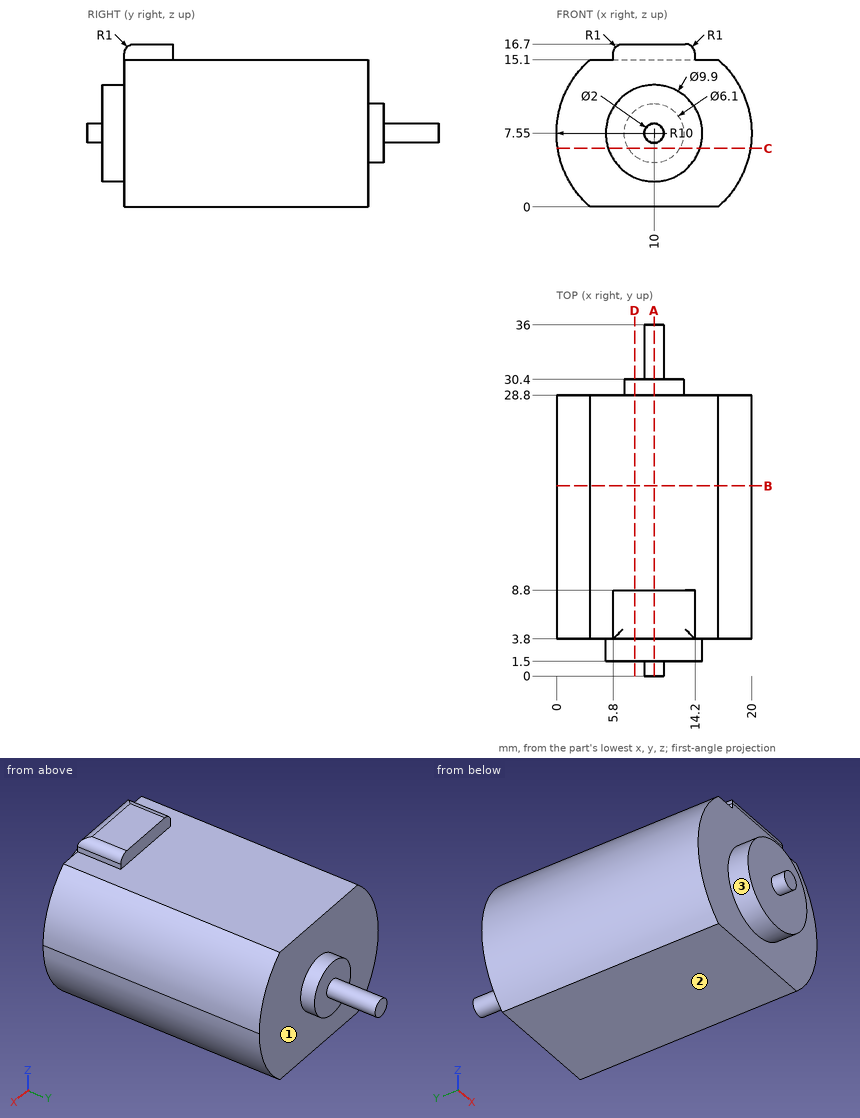
Print and shaded views of the part. All mm, measured from the part's lowest x, y and z. A direction names the side the tool comes from. Give positions to 0.01 mm unless a question says otherwise; leave off trailing zeros. Loops run counter-clockwise (first coordinate to the right, second up) from the corner with the lowest first, then second, coordinate; pieces in that order, holes last. Notation, with made-up numbers: (88.5, 34) -> (100.5, 34) arc R18 ccw to (100.5, 67) -> close; hole circle Ø3 at (28, 72). An arc over 180 degrees is marked (long way). Use a Markdown table: item, result.
1. Wall check: L1, parallel to Y at x = 6.25, z = 14.25; L2, parallel to X at y = 35.5, z = 7.5; L3, parallel to Z at x = 7.75, y = 25.5. Give the ranges that are in metal, low to high. Write a range as [from, to].
Check result:
| item | result |
|---|---|
| L1 | y = [3.8, 28.8] |
| L2 | x = [9, 11] |
| L3 | z = [0, 15.1] |
2. Which spindle directions (+Z, -Z, +X, -X, +Y, -Y) get a long thin tool onto all of the face, cutting with end or side? Do the marked faces 1, 2 and 3. Say none if no direction does.
Check result:
| item | result |
|---|---|
| face 1 | +Y |
| face 2 | -Z, +X, -X, +Y, -Y |
| face 3 | -Y |
3. Slice it at C-C (z = 6). List the corners of the cut face in (x, y), plus the area to 3 significant figures.
Check result:
| item | result |
|---|---|
| outline | (0.12, 3.8) -> (5.3, 3.8) -> (5.3, 1.5) -> (14.7, 1.5) -> (14.7, 3.8) -> (19.88, 3.8) -> (19.88, 28.8) -> (12.63, 28.8) -> (12.63, 30.4) -> (7.37, 30.4) -> (7.37, 28.8) -> (0.12, 28.8) -> close |
| area | 524 mm^2 |
4. Slice it at A-A (x = 10). List the corners of the cut face in (y, z).
Check result:
| item | result |
|---|---|
| outline | (0, 6.55) -> (1.5, 6.55) -> (1.5, 2.6) -> (3.8, 2.6) -> (3.8, 0) -> (28.8, 0) -> (28.8, 4.5) -> (30.4, 4.5) -> (30.4, 6.55) -> (36, 6.55) -> (36, 8.55) -> (30.4, 8.55) -> (30.4, 10.6) -> (28.8, 10.6) -> (28.8, 15.1) -> (8.8, 15.1) -> (8.8, 16.7) -> (4.8, 16.7) arc R1 ccw to (3.8, 15.7) -> (3.8, 12.5) -> (1.5, 12.5) -> (1.5, 8.55) -> (0, 8.55) -> close |
5. Slice it at B-B (y = 19.5). List the corners of the cut face in (x, z).
Check result:
| item | result |
|---|---|
| outline | (3.44, 0) -> (16.56, 0) arc R10 ccw to (16.56, 15.1) -> (3.44, 15.1) arc R10 ccw to start |
6. Slice it at D-D (x = 8). List the corners of the cut face in (y, z), plus the area to 3 significant figures.
Check result:
| item | result |
|---|---|
| outline | (1.5, 3.02) -> (3.8, 3.02) -> (3.8, 0) -> (28.8, 0) -> (28.8, 5.25) -> (30.4, 5.25) -> (30.4, 9.85) -> (28.8, 9.85) -> (28.8, 15.1) -> (8.8, 15.1) -> (8.8, 16.7) -> (4.8, 16.7) arc R1 ccw to (3.8, 15.7) -> (3.8, 12.08) -> (1.5, 12.08) -> close |
| area | 413 mm^2 |
7. Flat gauge pins, fed straight in: pin 1 (1 mm diameter, centred on y = 19.5, z = 1.5, fed in from +X); pin 2 (3 mm diameter, centred on y = 14, z = 14.5, fed in from -X); pin 3 (8 mm diameter, centred on x = 17.5, y = 17, fed in from +Z). Where does each tip first touch, or does it go through?
Check result:
| item | result |
|---|---|
| pin 1 | stops at x = 18.32 |
| pin 2 | stops at x = 1.62 |
| pin 3 | stops at z = 15.1 |
